Check sheet for the modelled part. Datum: model origin and axes. Units: mm. A direction names the side the tool comes from. Round coordinates to 2 decimals unless told otherwise and drop trailing zeros. Loops run counter-clockwise (first coordinate to the right, second up) from the corner with the lowest first, then second, coordinate; pieces in that order, holes last. Notation, with made-up numbers: (32.5, -9.75) - (38.5, -9.75) arc R19 cw to (38.5, 5.25) - close; hole circle Ø5 at (87, 57.5). An arc over 180 degrees is marked (long way). Put each result on its own line as item: value. Start each with the question number.
Item 1: Tool access check on faces 1 (the flat face through (4.59, 34.15, -1.31)), 2 (the cylindrical face through (27.699, 27.178, -4.856)). Record the directions out of +Z, -Z, +X, -X, +Y, -Y that give a thin tool (end or side, any length) a straight path to the whole face; none if there is none.
Item 2: Section check A-A, the plane x = 19.5. Record the cut outline in (y, z).
Item 3: Material ranges on line 1 along Y through (x, z) = (23, -2.5); line 2 along Y through (x, z) = (11.25, -4); line 3 along X through (y, z) = (17, -6.5), recorded low to high.
Item 4: Gauge pin test, flat ends, axial feed: pin 1 Ø1 at (x, z) = (23, -2.5) entering from +Y; pin 2 Ø1.1 at (x, z) = (7.5, -1.5) entering from +Y; pin 3 Ø3 at (y, z) = (24, -6) entering from +X. Record the tip position at first contact, or that the pin passes through.
from build123d import *

# Parameters (mm, degrees)
EXTRUDE_1_DEPTH        = 28
FILLET_1_R             = 1
SWEEP_1_PROFILE_R      = 0.7
PATTERN_LINEAR_1_COUNT = 2
PATTERN_LINEAR_1_PITCH = 2.5


with BuildPart() as part:
    # 草图1 → 凸台-拉伸1 (new body)
    with BuildSketch(Plane(origin=(0, 0, 0), x_dir=(0, 0, -1), z_dir=(1, 0, 0))):
        Polygon((0, 0), (0, 31), (3, 31), (7, 24), (7, 0), align=None)
    extrude(amount=EXTRUDE_1_DEPTH)

    # 圆角1
    fillet_1_edges = [part.edges().sort_by_distance(p)[0] for p in [
        (28, 27.5, -5),
        (28, 31, -1.5),
        (28, 15.5, 0),
        (28, 0, -3.5),
        (0, 15.5, 0),
        (0, 31, -1.5),
        (0, 27.5, -5),
        (0, 12, -7),
        (0, 0, -3.5),
        (28, 12, -7),
        (14, 0, 0),
        (14, 31, 0),
        (14, 31, -3),
        (14, 24, -7),
        (14, 0, -7),
    ]]
    fillet(fillet_1_edges, radius=FILLET_1_R)

    # 扫描1: sweep along a path in 草图2
    with BuildLine(Plane.XY.offset(-1.3)) as sweep_1_path:
        ThreePointArc((4.647498894, 28.922984251), (3.714501518, 31.52399057), (4.597001461, 34.142561139))
    # 扫描1 profile (on start of the path) → 扫描1 (sweep)
    with BuildSketch(Plane(origin=(4.647498894, 28.922984251, -1.3), x_dir=(0.778109821, 0.628128256, 0), z_dir=(-0.628128256, 0.778109821, 0))):
        Circle(SWEEP_1_PROFILE_R)
    sweep_1 = sweep(path=sweep_1_path.line)

    # 阵列(线性)1: 扫描1 ×2
    with Locations(*[(i * PATTERN_LINEAR_1_PITCH, 0, 0) for i in range(1, PATTERN_LINEAR_1_COUNT)]):
        add(sweep_1)


solid = part.part
Check result:
1. face 1: +Z, -Z, +Y
1. face 2: -Z, +X, +Y
2. outline: (0, -6) arc R1 ccw to (1, -7) - (23.73, -7) arc R1 ccw to (24.23, -6.87) - (30.5, -3.29) arc R1 ccw to (31, -2.42) - (31, -1) arc R1 ccw to (30, 0) - (1, 0) arc R1 ccw to (0, -1) - close
3. line 1: 0 to 31
3. line 2: 0 to 29.25
3. line 3: 0.13 to 27.87
4. pin 1: y = 31
4. pin 2: y = 34.26
4. pin 3: x = 28
